Part model, mm, in its own coordinate system. Face numbers are marked on the shaded views. A direction names the side the tool comes from. Give positions to 0.01 mm unless a question says otherwise; leave off trailing zeros. Order: outer loops, then holes, each group sorted by start corner. A loop starts at its lowest first (then second) coordinate and runs counter-clockwise, first axis right, second up. Notation, with made-up numbers: (49, -9.5) - (73, -9.5) arc R23 ccw to (73, 24.5) - close; hole circle Ø1 at (22.5, -33.5). An arc over 180 degrees is marked (long way). One line per item, written item: value.
```python
from build123d import *

# Parameters (mm, degrees)
F1_DEPTH = 11.25
F2_R     = 1.75
F3_DEPTH = 15
F4_R     = 3
F5_DEPTH = 6.3
F6_R     = 3.5
F7_DEPTH = 7.2
F8_R     = 1
F9_DEPTH = 15
F11_R    = 0.2


# Not quite as in the source:
# - a fillet or chamfer that OpenCascade refuses, or shapes differently, is made with other operations: its cross-section is extruded or revolved along the edge and cut away or added


with BuildPart() as f1:
    # F0 (on Front) → F1 (new body)
    with BuildSketch(Plane.XZ):
        with BuildLine():
            Line((6.25, 0), (6.25, 4.2355637169))
            ThreePointArc((6.25, 4.2355637169), (0, 7.55), (-6.25, 4.2355637169))
            Line((-6.25, 4.2355637169), (-6.25, -4.2355637169))
            ThreePointArc((-6.25, -4.2355637169), (0, -7.55), (6.25, -4.2355637169))
            Line((6.25, -4.2355637169), (6.25, 0))
        make_face()
    extrude(amount=F1_DEPTH)

    # F2 (on face) → F3 (cut)
    with BuildSketch(Plane.YZ.offset(6.25)):
        with Locations((-5.625, 0)):
            Circle(F2_R)
    extrude(amount=-F3_DEPTH, mode=Mode.SUBTRACT)

    # F4 (on face) → F5 (join)
    with BuildSketch(Plane(origin=(0, 0, 0), x_dir=(-1, 0, 0), z_dir=(0, 1, 0))):
        Circle(F4_R)
    extrude(amount=F5_DEPTH)

    # F6 (on face) → F7 (join)
    with BuildSketch(Plane.XZ.offset(11.25)):
        Circle(F6_R)
    extrude(amount=F7_DEPTH)

    # F8 (on face) → F9 (cut)
    with BuildSketch(Plane.YZ.offset(6.25)):
        with Locations((-14.3, 0)):
            Circle(F8_R)
    extrude(amount=-F9_DEPTH, mode=Mode.SUBTRACT)

    # F10: fillet of radius 3.5 on 1 edges, made by hand

    # F10_s1 → F10_t2 (revolve, cut)
    with BuildSketch(Plane.XY):
        with BuildLine():
            ThreePointArc((3.5, -14.95), (2.4748737342, -17.4248737342), (0, -18.45))
            Line((0, -18.45), (3.5, -18.45))
            Line((3.5, -18.45), (3.5, -14.95))
        make_face()
    revolve(axis=Axis((0, -18.45, 0), (0, -1, 0)), mode=Mode.SUBTRACT)

    # F11
    f11_edges = [f1.edges().sort_by_distance(p)[0] for p in [
        (3, 6.3, 0),
        (0, 0, 7.55),
        (6.25, 0, 0),
        (0, 0, -7.55),
        (-6.25, 0, 0),
        (0, -11.25, 7.55),
        (0, -11.25, -7.55),
        (-6.25, -11.25, 0),
        (6.25, -11.25, 0),
    ]]
    fillet(f11_edges, radius=F11_R)


solid = f1.part
```
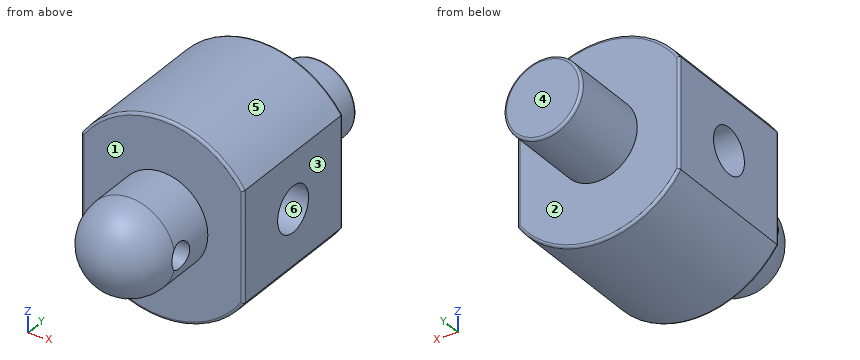
1) Cut at B-B, the plane x = 0. Give the cut face in (y, z) (3 decimals), then the cut area to 3 significant figures.
Outcome:
outline: (-14.95, -3.5) - (-11.25, -3.5) - (-11.25, -7.35) arc R0.2 ccw to (-11.05, -7.55) - (-0.2, -7.55) arc R0.2 ccw to (0, -7.35) - (0, -3) - (6.1, -3) arc R0.2 ccw to (6.3, -2.8) - (6.3, 2.8) arc R0.2 ccw to (6.1, 3) - (0, 3) - (0, 7.35) arc R0.2 ccw to (-0.2, 7.55) - (-11.05, 7.55) arc R0.2 ccw to (-11.25, 7.35) - (-11.25, 3.5) - (-14.95, 3.5) arc R3.5 ccw to start; hole circle Ø2 at (-14.3, 0); hole circle Ø3.5 at (-5.625, 0)
area: 240 mm^2
2) Mould opens along Z. For the marked faces 4, 5 and 6 say: released by +Z, released by -Z, zero draft, split by the parting line, or undercut.
Outcome:
face 4: zero draft
face 5: released by +Z
face 6: undercut
3) Cut at D-D, the plane y = 1.25. Give the cut face in (x, z).
Outcome:
outline: circle Ø6 at (0, 0)
4) Cut at C-C, the plane y = -14.3. Give the cut face in (x, z).
Outcome:
outline: (-3.35, -1) arc R3.5 ccw to (3.35, -1) - close; (-3.35, 1) - (3.35, 1) arc R3.5 ccw to start
5) Pin check, flat tips, straight feed: pin 1 (2 mm diameter, centred on x = -2.5, y = -5.5, fed in from -Z); pin 2 (3 mm diameter, centred on x = 4.5, y = 0.5, fed in from -Z); pin 3 (2 mm diameter, centred on x = 4, z = 4, fed in from +Y). Stop position of each tip, or through.
Outcome:
pin 1: stops at z = -7.4
pin 2: stops at z = -6.86
pin 3: stops at y = 0
6) Cut at A-A, the plane z = 0. Give the cut face in (x, y) (3 decimals), then the cut area to 3 significant figures.
Outcome:
outline: (-6.25, -11.05) arc R0.2 ccw to (-6.05, -11.25) - (-3.5, -11.25) - (-3.5, -13.3) - (3.5, -13.3) - (3.5, -11.25) - (6.05, -11.25) arc R0.2 ccw to (6.25, -11.05) - (6.25, -7.375) - (-6.25, -7.375) - close; (-6.25, -3.875) - (6.25, -3.875) - (6.25, -0.2) arc R0.2 ccw to (6.05, 0) - (3, 0) - (3, 6.1) arc R0.2 ccw to (2.8, 6.3) - (-2.8, 6.3) arc R0.2 ccw to (-3, 6.1) - (-3, 0) - (-6.05, 0) arc R0.2 ccw to (-6.25, -0.2) - close; (-3.482, -15.3) arc R3.5 ccw to (3.482, -15.3) - close
area: 166 mm^2
7) Which spindle directions (+Z, -Z, +X, -X, +Y, -Y) get a long thin tool onto all of the face, cutting with end or side? Do the marked faces 1, 2 and 3. Say none if no direction does.
Outcome:
face 1: -Y
face 2: +Y
face 3: +Z, -Z, +X, +Y, -Y
8) Drill centre lines: line 1 along Y through (x, z) = (-0.5, 6.25); line 2 along Z through (x, y) = (2.25, -14.5); line 3 along Z through (x, y) = (-0.25, -10). Where is each one in solid material? Low to high. Write a range as from..to.
Outcome:
line 1: y = -11.25..0
line 2: z = -2.68..-0.98, 0.98..2.68
line 3: z = -7.55..7.55
